Geometry check sheet. Reference: drawing and pictorial views, mm from the part's lowest x, y, z. Coordinates: 2 decimals unless noted, no trailing zeros. Order: outer loops, then holes, each group sorted by start corner. A loop starts at its lowest first (then second) coordinate and runs counter-clockwise, first axis right, second up. Notation, with made-up numbers: (52.25, 26.5) -> (92.25, 26.5) arc R26 cw to (92.25, 48.5) -> close; hole circle Ø1 at (79.25, 28.25). An arc over 180 degrees is marked (long way). Use CSV: the item, a comma, the result in double quotes. Start each with the question number.
1) Sectioned sample at A-A on x = 186.5. Record the boundary of the cut face in (y, z).
2) Sectioned sample at C-C on z = 21.5. Record the boundary of the cut face in (x, y).
3) Sectioned sample at B-B on y = 112. Record the boundary of the cut face in (x, z), then the cut area to 3 significant figures.
4) Scan lines: line 1 along X through (y, z) = (132, 14.25); line 2 along Y through (x, z) = (179, 2.5). Record each from-to range of solid material in increasing order.
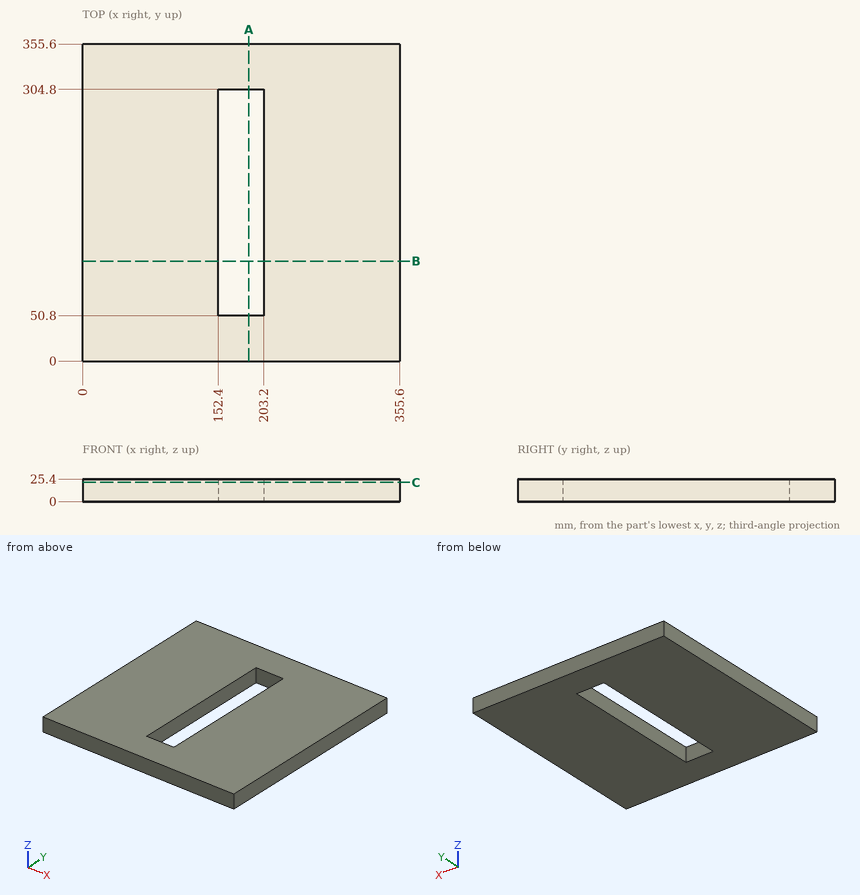
Answers follow:
1,outline,"(0, 0) -> (50.8, 0) -> (50.8, 25.4) -> (0, 25.4) -> close; (304.8, 0) -> (355.6, 0) -> (355.6, 25.4) -> (304.8, 25.4) -> close"
2,outline,"(0, 0) -> (355.6, 0) -> (355.6, 355.6) -> (0, 355.6) -> close; hole (152.4, 50.8) -> (203.2, 50.8) -> (203.2, 304.8) -> (152.4, 304.8) -> close"
3,outline,"(0, 0) -> (152.4, 0) -> (152.4, 25.4) -> (0, 25.4) -> close; (203.2, 0) -> (355.6, 0) -> (355.6, 25.4) -> (203.2, 25.4) -> close"
3,area,"7,740 mm²"
4,line 1,"x = 0 to 152.4, 203.2 to 355.6"
4,line 2,"y = 0 to 50.8, 304.8 to 355.6"
